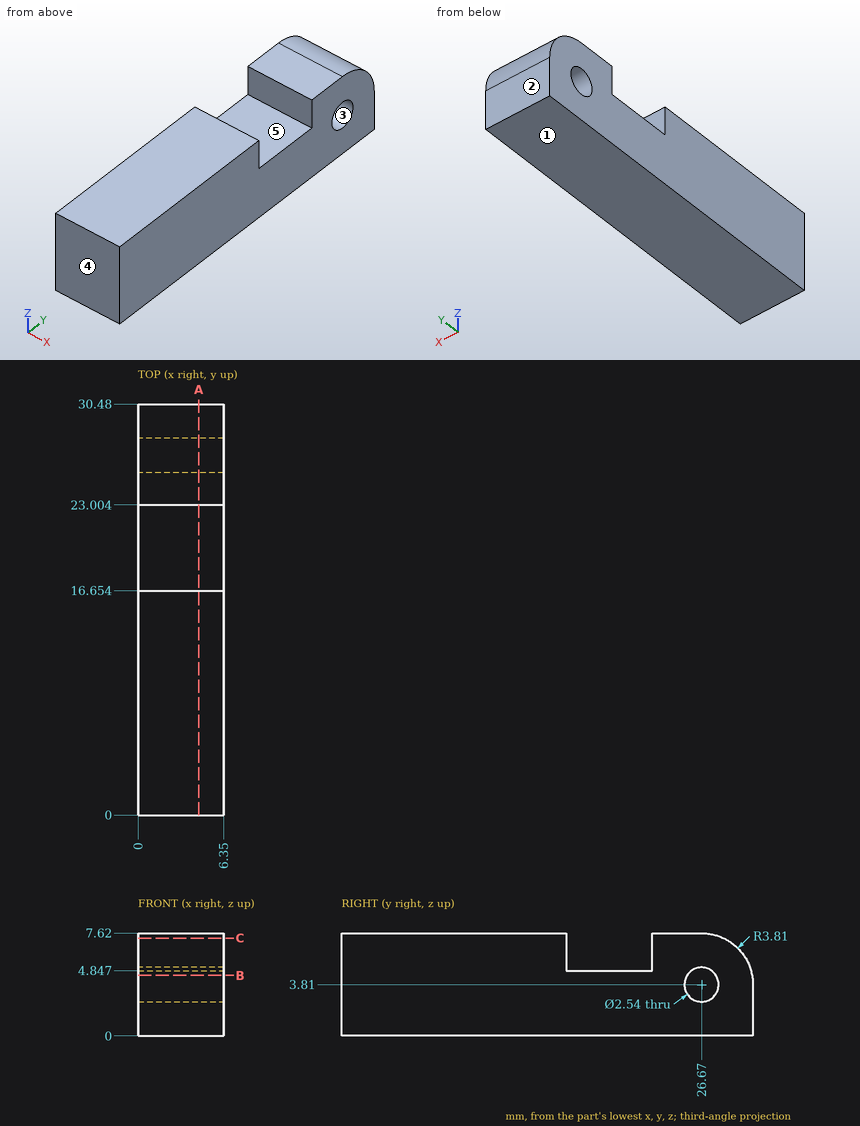
Geometry: see drawing. Coordinates: mm, zero at the bounding-box minimum. A direction names the side the tool comes from. Give positions to 0.01 mm unless a question says otherwise; leave off trailing zeros. Write each loop counter-clockwise with the first axis right and the second up, starting at its lowest first coordinate (ties: lowest second). Pieces come first, ordered by that corner, then holes. Notation, with made-up numbers: M 67,-15 L 117,-15 A26 cw 117,8 Z; hole C 9,28.5 d4. An arc over 180 degrees is marked long. Return JSON: item names as keys, results as strings. Group by question number.
1) Set-up query: the marked faces 4 and 5. Return all of +Z, -Z, +X, -X, +Y, -Y with unobstructed straight access to the full face (end or side cutting, diameter ignored); none if empty.
2) First-contact query: pin 1 Ø2 at (y, z) = (4, 5.5) entering from -X; pin 2 Ø1.4 at (x, z) = (2, 6) entering from +Y. Flat tips, straight axial feed; report the tip coordinate or a pass-through.
3) Ray query, L1, parallel to Y at x = 2.5, z = 3.81; L2, parallel to Y at x = 2, z = 3; L3, parallel to Z at x = 5, y = 21.5. Return the intervals inside material, ascending.
4) Cut plane B-B, the plane z = 4.5. Output: boundary loops of the cut face in (x, y), then the cut area to 3 significant figures.
5) Draft query along Y for the marked faces 1, 2 and 3. Return one class per face: released by +Y, released by -Y, zero draft, split by the parting line, or undercut.
6) Cut plane A-A, the plane x = 4.5. Output: boundary loops of the cut face in (y, z).
7) Cut plane C-C, the plane z = 7.25. Output: boundary loops of the cut face in (x, y).
Data:
{
 "1": {"face 4": "+Z, -Z, +X, -X, -Y", "face 5": "+Z, +X, -X"},
 "2": {"pin 1": "stops at x = 0", "pin 2": "stops at y = 30.18"},
 "3": {"L1": "y = 0 to 25.4, 27.94 to 30.48", "L2": "y = 0 to 25.69, 27.65 to 30.48", "L3": "z = 0 to 4.85"},
 "4": {"outline": "M 0,0 L 6.35,0 L 6.35,25.6 L 0,25.6 Z; M 0,27.74 L 6.35,27.74 L 6.35,30.42 L 0,30.42 Z", "area": "180 mm²"},
 "5": {"face 1": "zero draft", "face 2": "released by +Y", "face 3": "undercut"},
 "6": {"outline": "M 0,0 L 30.48,0 L 30.48,3.81 A3.81 ccw 26.67,7.62 L 23,7.62 L 23,4.85 L 16.65,4.85 L 16.65,7.62 L 0,7.62 Z; hole C 26.67,3.81 d2.54"},
 "7": {"outline": "M 0,0 L 6.35,0 L 6.35,16.65 L 0,16.65 Z; M 0,23 L 6.35,23 L 6.35,28.31 L 0,28.31 Z"}
}
